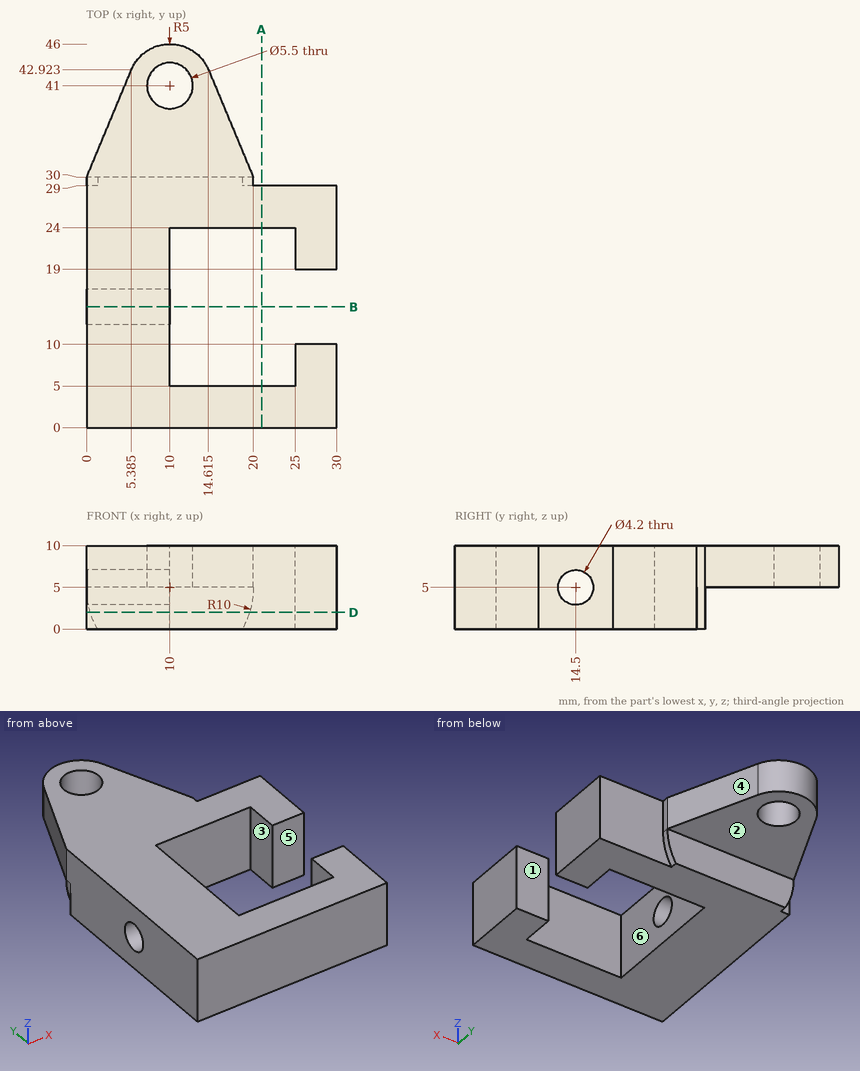
For this review, use the dimensioned drawing (mm, ordinates from the lowest corner) and the shaded views. A direction names the side the tool comes from. Coordinates: 2 decimals unless noted, no trailing zeros. Write each loop counter-clockwise with the first axis right and the second up, starting at its lowest first coordinate (ties: lowest second). Pieces come first, ordered by that corner, then holes. Notation, with made-up numbers: (-26, 40) - (17, 40) arc R19 cw to (17, 69) - close; hole circle Ø2 at (-26, 11.25). An arc over 180 degrees is marked (long way). Answer as a JSON object with one key per item and string values. Group by question number.
1. To check wall thickness, follow probe 1 along Z at (x, y) = (5, 14.5); probe 2 along Y at (x, z) = (12.5, 8) (1 decimal); probe 3 along Y at (x, z) = (20, 1.5). State the ranges of each line that lie inside material, in increasing order.
2. Clearance check with flat-ended pins moving along their axes: pin 1 Ø3.5 at (x, y) = (10, 41) entering from +Z; pin 2 Ø5.5 at (x, z) = (7, 3) entering from +Y (1 decimal); pin 3 Ø5 at (x, z) = (14.5, 3.5) entering from +Y; pin 4 Ø4 at (x, z) = (28.5, 4) entering from +Y. State where each tip first meets the part, or that it passes through.
3. Add section A-A (x = 21). Give the boundary of the cut face in (y, z).
4. Add section D-D (z = 2). Give the boundary of the cut face in (x, y).
5. Machinability: for the marked faces 1, 2 and 3, which of the approach directions +Z, -Z, +X, -X, +Y, -Y give a long, thin tool a straight path to every point of the face, cutting with its end or side? Answer none if there is none.
6. Mouldability with a two-part tool opening along X and no side actions: class the marked faces 4, 5 and 6 as pulls with the +X half, pulls with the -X half, needs draft (parallel to the pull), parting line crosses it, or undercut.
7. Add section B-B (y = 14.5). Give the boundary of the cut face in (x, z).
Findings:
{
 "1": {"probe 1": "0 to 2.9, 7.1 to 10", "probe 2": "0 to 5, 24 to 39.9, 42.1 to 45.3", "probe 3": "0 to 5, 24 to 29"},
 "2": {"pin 1": "through", "pin 2": "y = 45.9", "pin 3": "y = 45.33", "pin 4": "y = 29"},
 "3": {"outline": "(0, 0) - (5, 0) - (5, 10) - (0, 10) - close; (24, 0) - (29, 0) - (29, 10) - (24, 10) - close"},
 "4": {"outline": "(0, 0) - (30, 0) - (30, 10) - (25, 10) - (25, 5) - (10, 5) - (10, 24) - (25, 24) - (25, 19) - (30, 19) - (30, 29) - (19.54, 29) - (19.54, 30) - (0.46, 30) - (0.46, 29) - (0, 29) - close"},
 "5": {"face 1": "+Z, -Z, +X", "face 2": "-Z, +X, -X, +Y", "face 3": "+Z, -Z"},
 "6": {"face 4": "pulls with the +X half", "face 5": "needs draft", "face 6": "undercut"},
 "7": {"outline": "(0, 0) - (10, 0) - (10, 2.9) - (0, 2.9) - close; (0, 7.1) - (10, 7.1) - (10, 10) - (0, 10) - close"}
}
